Verification items for the finished model (mm, model axes). Face numbers are marked on the shaded views. A direction names the side the tool comes from. Round coordinates to 2 decimals unless told otherwise and drop trailing zeros. Order: outer loops, then holes, each group sorted by start corner. A loop starts at its lowest first (then second) coordinate and runs counter-clockwise, first axis right, second up. Notation, with made-up numbers: (67, -26.75) -> (86, -26.75) arc R19 ccw to (86, -5.75) -> close; hole circle Ø9 at (-6, 18). An arc over 180 degrees is marked (long way). Return JSON: item names as keys, results as strings. Group by question number.
Item 1: Sectioned sample at A-A on z = 7. Record the cut outline in (x, y), plus the area to 3 significant figures.
Item 2: Sectioned sample at C-C on x = 3. Record the cut outline in (y, z), plus the area to 3 significant figures.
Item 3: Sectioned sample at B-B on z = 12. Record the cut outline in (x, y), plus the area to 3 significant figures.
Item 4: Access from +Z, -Z, +X, -X, +Y, -Y to the whole of each face (thin tool, end or side, straight path). Record for the marked faces 4 and 5.
Item 5: Scan lines: probe 1 along Y at (x, z) = (0, 6.5); probe 2 along Z at (x, y) = (1.5, -1.75); probe 3 along Y at (x, z) = (-1, 6). Record each from-to range of solid material in increasing order. Write a range as from..to.
Item 6: Depth check by flat-ended pin: pin 1 Ø2 at (x, y) = (0, 0) entering from -Z. Enter the tip coordinate at first touch or a pass-through.
Item 7: Draft check along X on the marked faces 1, 2 and 3. Enter one of: pulls with the +X half, pulls with the -X half, needs draft (parallel to the pull), parting line crosses it, or undercut.
Item 8: Sectioned sample at D-D on y = -2.5. Record the cut outline in (x, z).
```python
from build123d import *

# Parameters (mm, degrees)
BOSS_EXTRUDE1_DEPTH       = 25
SKETCH2_R                 = 2
BOSS_EXTRUDE2_DEPTH       = 6
M4X0_7_TAPPED_HOLE1_D     = 3.3
M4X0_7_TAPPED_HOLE1_DEPTH = 10.1
M4X0_7_TAPPED_HOLE1_TIP   = 0.991420021


with BuildPart() as part:
    # Sketch1 → Boss-Extrude1 (new body)
    with BuildSketch(Plane.XY):
        Polygon((3.464101615, 0), (1.732050808, 3), (-1.732050808, 3), (-3.464101615, 0), (-1.732050808, -3), (1.732050808, -3), align=None)
    extrude(amount=BOSS_EXTRUDE1_DEPTH)

    # Sketch2 → Boss-Extrude2 (add)
    with BuildSketch(Plane.XY.offset(25)):
        Circle(SKETCH2_R)
    extrude(amount=BOSS_EXTRUDE2_DEPTH)

    # M4x0.7 Tapped Hole1
    with Locations(Plane(origin=(0, 0, 0), x_dir=(-1, 0, 0), z_dir=(0, 0, -1))):
        with Locations((0, 0)):
            Hole(M4X0_7_TAPPED_HOLE1_D / 2, depth=M4X0_7_TAPPED_HOLE1_DEPTH)
            with Locations((0, 0, -(M4X0_7_TAPPED_HOLE1_DEPTH + M4X0_7_TAPPED_HOLE1_TIP / 2))):  # 118° drill point
                Cone(0, M4X0_7_TAPPED_HOLE1_D / 2, M4X0_7_TAPPED_HOLE1_TIP, mode=Mode.SUBTRACT)


solid = part.part
```
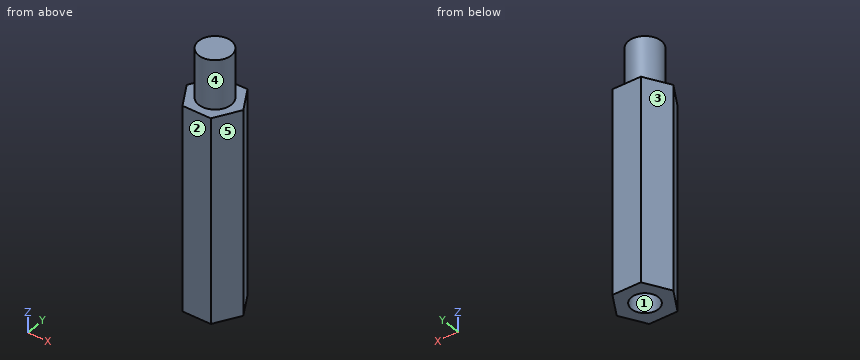
Recorded:
{
 "1": {"outline": "(-3.46, 0) -> (-1.73, -3) -> (1.73, -3) -> (3.46, 0) -> (1.73, 3) -> (-1.73, 3) -> close; hole circle Ø3.3 at (0, 0)", "area": "22.6 mm²"},
 "2": {"outline": "(-0.8, 0) -> (0.8, 0) -> (0.8, 25) -> (-0.8, 25) -> close", "area": "40.2 mm²"},
 "3": {"outline": "(-3.46, 0) -> (-1.73, -3) -> (1.73, -3) -> (3.46, 0) -> (1.73, 3) -> (-1.73, 3) -> close", "area": "31.2 mm²"},
 "4": {"face 4": "+Z", "face 5": "+Z, -Z, +X, -Y"},
 "5": {"probe 1": "-3..-1.65, 1.65..3", "probe 2": "0..25", "probe 3": "-3..-1.31, 1.31..3"},
 "6": {"pin 1": "z = 10.49"},
 "7": {"face 1": "undercut", "face 2": "needs draft", "face 3": "pulls with the -X half"},
 "8": {"outline": "(-2.02, 0) -> (2.02, 0) -> (2.02, 25) -> (-2.02, 25) -> close"}
}
